Geometry check sheet. Reference: the model listing, model coordinates, mm. Round coordinates to 2 decimals unless told otherwise and drop trailing zeros. Order: outer loops, then holes, each group sorted by start corner. A loop starts at its lowest first (then second) coordinate and runs counter-clockwise, first axis right, second up.
(1) Cross-section at B-B on y = -2.35. Count the separate pieces of the cut face and the enclosed holes in it, and give its area (3 significant figures).
(2) Draft check along X on faces 1 (the face through (-69.766, -1.503, -4.354)), 2 (the face through (-186.67, -1.5, 44.36)), 3 (the face through (37.531, -1.503, -91.115)). Enter one of: pulls with the +X half, pulls with the -X half, needs draft (parallel to the pull), parting line crosses it, or undercut.
(3) Cross-section at C-C on z = -24. Enter the section's corners in (x, y).
(4) Gauge pin test, flat end, axial feed: P1, Ø10.5, axis at x = -38.52, z = -10.08, coming from the +Y side (1 decimal). Record the tip position at first contact, or that the pin passes through.
(5) Cross-section at A-A on x = -20. Enter the section's corners in (y, z).
(6) Thickness scan on L1, parallel to X at y = -1.8, z = -89.5; L2, parallel to Z at x = -161.5, y = -1.5; L3, parallel to X at y = -0.6, z = -88. Record the ranges inside material, lowest first.
from build123d import *

# Parameters (mm, degrees)
F0_R     = 4.7625
F0_R_2   = 5.953125
F0_R_3   = 19.05
F1_DEPTH = 3.048


with BuildPart() as f1:
    # F0 (on Front) → F1 (new body)
    with BuildSketch(Plane.XZ):
        with BuildLine():
            ThreePointArc((-180.010916, 47.074063), (-186.746108, 44.284255), (-189.535916, 37.549063))
            Line((-189.535916, 37.549063), (-189.535916, -95.800937))
            ThreePointArc((-189.535916, -95.800937), (-186.746108, -102.536129), (-180.010916, -105.325937))
            Line((-180.010916, -105.325937), (8.377442, -105.325937))
            ThreePointArc((8.377442, -105.325937), (10.43903, -105.100157), (12.402881, -104.433519))
            Line((12.402881, -104.433519), (33.564523, -94.565683))
            ThreePointArc((33.564523, -94.565683), (37.572388, -91.05088), (39.064084, -85.933102))
            Line((39.064084, -85.933102), (39.064084, 37.549063))
            ThreePointArc((39.064084, 37.549063), (36.274276, 44.284255), (29.539084, 47.074063))
            Line((29.539084, 47.074063), (-180.010916, 47.074063))
        make_face()
        with Locations((-164.920668, -91.929214)):
            Circle(F0_R, mode=Mode.SUBTRACT)
        with Locations((-76.149133, -91.929214)):
            Circle(F0_R_2, mode=Mode.SUBTRACT)
        with Locations((-29.71804, -75.029679)):
            Circle(F0_R_3, mode=Mode.SUBTRACT)
        with Locations((16.713054, -58.130143)):
            Circle(F0_R_2, mode=Mode.SUBTRACT)
        with Locations((-137.346853, -10.075937)):
            Circle(F0_R_2, mode=Mode.SUBTRACT)
        with Locations((-87.935916, -10.075937)):
            Circle(F0_R_3, mode=Mode.SUBTRACT)
        with Locations((-164.920668, 29.595656)):
            Circle(F0_R, mode=Mode.SUBTRACT)
        with Locations((-38.524978, -10.075937)):
            Circle(F0_R_2, mode=Mode.SUBTRACT)
        with Locations((16.713054, 29.595656)):
            Circle(F0_R, mode=Mode.SUBTRACT)
    extrude(amount=F1_DEPTH)


solid = f1.part
Found:
1. separate pieces: 1
1. enclosed holes: 9
1. area: 31,600 mm2
2. face 1: undercut
2. face 2: pulls with the -X half
2. face 3: pulls with the +X half
3. outline: (-189.54, -3.05) - (-100.94, -3.05) - (-100.94, 0) - (-189.54, 0) - close; (-74.94, -3.05) - (39.06, -3.05) - (39.06, 0) - (-74.94, 0) - close
4. P1: passes through
5. outline: (-3.05, -105.33) - (0, -105.33) - (0, -91.41) - (-3.05, -91.41) - close; (-3.05, -58.64) - (0, -58.64) - (0, 47.07) - (-3.05, 47.07) - close
6. L1: x = -189.54 to -169.02, -160.82 to -81.58, -70.71 to -42.11, -17.33 to 38.37
6. L2: z = -105.33 to -95.24, -88.62 to 26.28, 32.91 to 47.07
6. L3: x = -189.54 to -167.61, -162.23 to -80.62, -71.68 to -43.67, -15.77 to 38.84
